```python
from build123d import *

# Parameters (mm, degrees)
EXTRUDE_1_DEPTH     = 500
SKETCH_2_W          = 40
SKETCH_2_H          = 30
CUT_EXTRUDE_1_DEPTH = 504.189825016
SKETCH_3_W          = 40
SKETCH_3_H          = 30
CUT_EXTRUDE_2_DEPTH = 504.189825016


with BuildPart() as part:
    # Эскиз1 → Бобышка-Вытянуть1 (new body)
    with BuildSketch(Plane.XY):
        Polygon((0, 0), (0, 40), (4, 40), (4, 4), (40, 4), (40, 0), align=None)
    extrude(amount=EXTRUDE_1_DEPTH)

    # Эскиз2 → Вырез-Вытянуть1 (cut, through all)
    with BuildSketch(Plane.ZY):
        with Locations((20, 25)):
            Rectangle(SKETCH_2_W, SKETCH_2_H)
    extrude(amount=-CUT_EXTRUDE_1_DEPTH, mode=Mode.SUBTRACT)

    # Эскиз3 → Вырез-Вытянуть2 (cut, through all)
    with BuildSketch(Plane.ZY):
        with Locations((480, 25)):
            Rectangle(SKETCH_3_W, SKETCH_3_H)
    extrude(amount=-CUT_EXTRUDE_2_DEPTH, mode=Mode.SUBTRACT)


solid = part.part
```
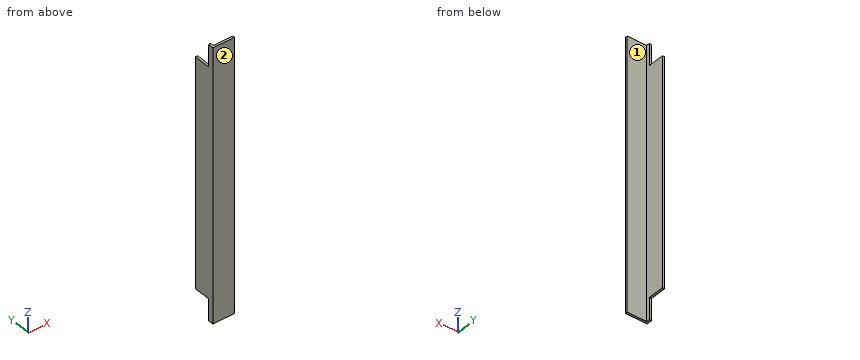
The listing builds one solid part. Answer for the finished solid, in the listing's coordinates (mm). Face numbers are marked on the shaded views. A direction names the side the tool comes from. Round coordinates to 2 decimals unless told otherwise and drop trailing zeros. Loops run counter-clockwise (first coordinate to the right, second up) from the corner with the lowest first, then second, coordinate; pieces in that order, holes last.
Q1. Section A-A, the plane z = 350.5 is taken. Determine the outline of the cut face in (x, y).
Q2. Section C-C, the plane x = 34.5 is taken. Determine the outline of the cut face in (y, z), then the cut area to 3 significant figures.
Q3. Given pin 1 Ø12 at (y, z) = (17.5, 246) entering from +X; pin 2 Ø11 at (x, z) = (20.5, 239.5) entering from +Y; pin 3 Ø1.2 at (x, y) = (1.5, 26.5) entering from -Z, each flat-ended and moving along its own axis, determine where each tip first touches the part or whether it passes through.
Q4. Section B-B, the plane y = 20 is taken. Determine the outline of the cut face in (x, z).
Q5. Find the intervals of material crossed by line 1 (X direction, y = 8, z = 446), in increasing order.
Q6. Which of the six approach directions +Z, -Z, +X, -X, +Y, -Y give full straight-line access (tool end or side, diameter ignored) to the marked faces 1 and 2?
Completed:
1. outline: (0, 0) - (40, 0) - (40, 4) - (4, 4) - (4, 40) - (0, 40) - close
2. outline: (0, 0) - (4, 0) - (4, 500) - (0, 500) - close
2. area: 2,000 mm2
3. pin 1: stops at x = 4
3. pin 2: stops at y = 4
3. pin 3: stops at z = 40
4. outline: (0, 40) - (4, 40) - (4, 460) - (0, 460) - close
5. line 1: x = 0 to 4
6. face 1: +Z, -Z, +X, +Y
6. face 2: +Z, -Z, +X, -X, -Y
